The listing builds one solid part. Answer for the finished solid, in the listing's coordinates (mm). A direction names the side the tool comes from. Give positions to 0.01 mm unless a question says otherwise; leave off trailing zeros. Loops run counter-clockwise (first coordinate to the right, second up) from the corner with the lowest first, then second, coordinate; pieces in that order, holes last. Notation, with made-up numbers: (34, 11) - (59, 11) arc R3 cw to (59, 16) - close; hole circle Ø3 at (26, 2.25). An arc over 180 degrees is marked (long way). Write item = value, one per line. Start each with the question number.
1) Flat-ended cylindrical pins translate along their axes: P1, Ø3.5, axis at x = 0.5, z = 16, coming from the +Y side; P2, Ø0.5, axis at y = 5.5, z = 28.5, coming from the +X side; P3, Ø5, axis at x = -1, z = 38.5, coming from the -Y side. Find the tip coordinate at first contact, or state that the pin passes through.
2) Consider probe 1 along Z at (x, y) = (-0.75, 6.5); probe 2 along X at (y, z) = (-2.75, 25.5); probe 3 along Y at (x, z) = (-0.25, 37.5). Determine where each line is inside the solid, lowest interval first.
3) The mould has two halves that part along Z. Classify faces 4 (the flat face through (3, -5, 46)), 5 (the flat face through (-1, 5.5, 23.7)), 6 (the flat face through (-3, 3, 0)): +Z half, -Z half, draft (parallel to the pull), parting line (faces both ways), or undercut.
4) The part is cut by section A-A on x = 0. Write down the section's boundary in (y, z), plus the area to 3 significant figures.
5) The part is cut by section B-B on z = 8.5. Write down the section's boundary in (x, y), plus the area to 3 significant figures.
6) Which of the six approach directions +Z, -Z, +X, -X, +Y, -Y give full straight-line access (tool end or side, diameter ignored) to faces 1 (the cylindrical face through (0.228, -5.495, 47.014)), 2 (the cylindrical face through (0, -6, 23)), 3 (the flat face through (0, 3.55, 25))?
from build123d import *

# Parameters (mm, degrees)
SKETCH_1_R                        = 6
EXTRUDE_1_DEPTH                   = 50
EXTRUDE_START                     = -2
SKETCH_2_R                        = 7
SKETCH_2_R_2                      = 6
EXTRUDE_2_DEPTH                   = 2
SKETCH_3_OUTSIDE_W                = 26.756
SKETCH_3_OUTSIDE_H                = 26.756
SKETCH_3_OUTSIDE_R                = 5.5
CUT_EXTRUDE_1_DEPTH               = 2
SKETCH_6_W                        = 2
SKETCH_6_H                        = 1
CUT_EXTRUDE_1_2_DEPTH             = 2
CUT_EXTRUDE_1_2_DIRECTION_2_REACH = 52.971


# Read off the part's stored shape, not the designer's step: M12 机械螺纹 螺柱1
with BuildPart() as part:
    # 草图1 → 凸台-拉伸1 (new body)
    with BuildSketch(Plane.XY):
        Circle(SKETCH_1_R)
        Polygon((4.099186911, 0), (2.049593456, 3.55), (-2.049593456, 3.55), (-4.099186911, 0), (-2.049593456, -3.55), (2.049593456, -3.55), align=None, mode=Mode.SUBTRACT)
    extrude(amount=EXTRUDE_1_DEPTH)

    # 草图2 → 凸台-拉伸2 (add)
    with BuildSketch(Plane.XY.offset(50).offset(EXTRUDE_START)):
        Circle(SKETCH_2_R)
        Circle(SKETCH_2_R_2, mode=Mode.SUBTRACT)
    extrude(amount=EXTRUDE_2_DEPTH)

    # 草图3 outside → Cut-Extrude 1 (cut)
    with BuildSketch(Plane(origin=(0, 0, 48), x_dir=(-1, 0, 0), z_dir=(0, 0, -1))):
        Rectangle(SKETCH_3_OUTSIDE_W, SKETCH_3_OUTSIDE_H)
        Circle(SKETCH_3_OUTSIDE_R, mode=Mode.SUBTRACT)
    extrude(amount=CUT_EXTRUDE_1_DEPTH, mode=Mode.SUBTRACT)

    # M12 机械螺纹 螺柱1 outline → M12 机械螺纹 螺柱1 (revolve, cut)
    with BuildSketch(Plane.XZ):
        Polygon((6, 0.947), (5.053, 0), (6, 0), align=None)
    revolve(axis=Axis((0, 0, 0), (0, 0, 1)), mode=Mode.SUBTRACT)

    # 草图6 → Cut-Extrude 1 2 (cut)
    with BuildSketch(Plane.XY):
        with Locations((0, 5.5)):
            Rectangle(SKETCH_6_W, SKETCH_6_H)
    extrude(amount=-CUT_EXTRUDE_1_2_DEPTH, mode=Mode.SUBTRACT)

    # Cut-Extrude 1 2 direction 2: up to this face of the body (flat: up to its plane)
    cut_extrude_1_2_direction_2_end = Plane(part.part.faces().sort_by_distance((5.697989899, 0, 48))[0])
    # 草图6 → Cut-Extrude 1 2 direction 2 (cut, up to the picked face)
    with BuildSketch(Plane.XY, mode=Mode.PRIVATE) as cut_extrude_1_2_direction_2_sk1:
        with Locations((0, 5.5)):
            Rectangle(SKETCH_6_W, SKETCH_6_H)
    cut_extrude_1_2_direction_2_tool1 = split(extrude(cut_extrude_1_2_direction_2_sk1.sketch, amount=CUT_EXTRUDE_1_2_DIRECTION_2_REACH, mode=Mode.PRIVATE), bisect_by=cut_extrude_1_2_direction_2_end, keep=Keep.BOTH, mode=Mode.PRIVATE)
    add(cut_extrude_1_2_direction_2_tool1.solids().sort_by(Axis((0, 5.5, 0), (0, 0, 1)))[0], mode=Mode.SUBTRACT)


solid = part.part
Answer below:
q1.P1 = 5.92
q1.P2 = 2.9
q1.P3 = -6
q2.probe_1 = 48 to 50
q2.probe_2 = -5.33 to -2.51, 2.51 to 5.33
q2.probe_3 = -5.99 to -3.55, 3.55 to 5
q3.face_4 = undercut
q3.face_5 = draft
q3.face_6 = -Z half
q4.outline = (-7, 48) - (-5.5, 48) - (-5.5, 46) - (-6, 46) - (-6, 0.95) - (-5.05, 0) - (-3.55, 0) - (-3.55, 50) - (-7, 50) - close; (3.55, 0) - (5, 0) - (5, 48) - (7, 48) - (7, 50) - (3.55, 50) - close
q4.area = 200 mm2
q5.outline = (-1, 5) - (-1, 5.92) arc R6 ccw (long way) to (1, 5.92) - (1, 5) - close; hole (-4.1, 0) - (-2.05, -3.55) - (2.05, -3.55) - (4.1, 0) - (2.05, 3.55) - (-2.05, 3.55) - close
q5.area = 67.5 mm2
q6.face_1 = none
q6.face_2 = -Z
q6.face_3 = +Z, -Z
